Could you check a few things on this model? Use its own coordinates, in mm. A direction names the side the tool comes from. Give positions to 0.01 mm unless a question says otherwise; leave off trailing zeros. Loops run counter-clockwise (first coordinate to the right, second up) from the corner with the lowest first, then second, coordinate; pieces in that order, holes last.
1. Imagine slicing it at D-D (y = 100). List the corners of the cut face in (x, z) for me, plus the area to 3 significant figures.
2. For faces 5 (the flat face through (-25.4, 66, 13)), 6 (the flat face through (25.4, 67, 13)), 7 (the flat face through (0, 27.5, 13)), which set-ups out of +Z, -Z, +X, -X, +Y, -Y let a thin tool reach every point of the face, with its end or its side?
3. For P1, Ø10, axis at y = 59, z = 18, coming from the -X side; P2, Ø3, axis at x = 7.5, z = 13.5, coming from the -Y side; P3, Ø5, axis at x = 17, y = 13.5, coming from the +Z side; P4, Ø0.8, axis at y = 27, z = 11.5, coming from the +X side, each with a flat end and sliding along its axis, tell me the tip position at first contact or that it passes through.
4. I need wall thicknesses on line 1 along X through (y, z) = (0, 14.25); line 2 along Y through (x, z) = (9, 8); line 3 along Y through (x, z) = (-11.25, 9.5). Which ranges of each line are inside material? Lowest first, please.
5. Thinking about a two-plate mould opening in Y: for faces 1 (the flat face through (0, 109.08, 13)), 2 (the cylindrical face through (-13.748, 65.11, 12.878)), 3 (the flat face through (0, 54, 0)), 4 (the flat face through (2.5, 26, 13)), which applies, +Y half, -Y half, draft (parallel to the pull), parting line (faces both ways), or undercut?
6. Imagine slicing it at B-B (x = 0). List the corners of the cut face in (y, z) for me.
7. Imagine slicing it at A-A (y = 0). List the corners of the cut face in (x, z) for me.
8. Imagine slicing it at C-C (z = 18.5). List the corners of the cut face in (x, y) for me.
```python
from build123d import *

# Parameters (mm, degrees)
SKETCH1_R           = 25
BOSS_EXTRUDE1_DEPTH = 25.4
SKETCH2_W           = 5
SKETCH2_H           = 27.5
CUT_EXTRUDE1_DEPTH  = 118.339581594
SKETCH3_R           = 2.5
CUT_EXTRUDE2_DEPTH  = 118.339581594


with BuildPart() as part:
    # Sketch1 → Boss-Extrude1 (new body)
    with BuildSketch(Plane.XY):
        with BuildLine():
            Line((-25.4, 24.079867109), (-25.4, 109.079867109))
            Line((-25.4, 109.079867109), (25.4, 109.079867109))
            Line((25.4, 109.079867109), (25.4, 24.079867109))
            ThreePointArc((25.4, 24.079867109), (0, -35), (-25.4, 24.079867109))
        make_face()
        Circle(SKETCH1_R, mode=Mode.SUBTRACT)
    extrude(amount=BOSS_EXTRUDE1_DEPTH)

    # Sketch2 → Cut-Extrude1 (cut, through all)
    with BuildSketch(Plane.XY.offset(25.4)):
        with Locations((0, 13.75)):
            Rectangle(SKETCH2_W, SKETCH2_H)
    extrude(amount=-CUT_EXTRUDE1_DEPTH, mode=Mode.SUBTRACT)

    # Sketch3 → Cut-Extrude2 (cut, through all)
    with BuildSketch(Plane.XY.offset(25.4)):
        with Locations((-11.25, 100)):
            Circle(SKETCH3_R)
        with Locations((11.25, 100)):
            Circle(SKETCH3_R)
        with Locations((11.25, 65)):
            Circle(SKETCH3_R)
        with Locations((-11.25, 65)):
            Circle(SKETCH3_R)
    extrude(amount=-CUT_EXTRUDE2_DEPTH, mode=Mode.SUBTRACT)


solid = part.part
```
Derived:
1. outline: (-25.4, 0) - (-13.75, 0) - (-13.75, 25.4) - (-25.4, 25.4) - close; (-8.75, 0) - (8.75, 0) - (8.75, 25.4) - (-8.75, 25.4) - close; (13.75, 0) - (25.4, 0) - (25.4, 25.4) - (13.75, 25.4) - close
1. area: 1,040 mm2
2. face 5: +Z, -Z, -X, +Y
2. face 6: +Z, -Z, +X, +Y
2. face 7: +Z, -Z
3. P1: stops at x = -25.4
3. P2: stops at y = -34.48
3. P3: passes through
3. P4: stops at x = 25.4
4. line 1: x = -35 to -25, 25 to 35
4. line 2: y = -33.82 to -23.32, 23.32 to 63.91, 66.09 to 98.91, 101.09 to 109.08
4. line 3: y = -33.14 to -22.33, 22.33 to 62.5, 67.5 to 97.5, 102.5 to 109.08
5. face 1: +Y half
5. face 2: undercut
5. face 3: draft
5. face 4: undercut
6. outline: (-35, 0) - (-25, 0) - (-25, 25.4) - (-35, 25.4) - close; (27.5, 0) - (109.08, 0) - (109.08, 25.4) - (27.5, 25.4) - close
7. outline: (-35, 0) - (-25, 0) - (-25, 25.4) - (-35, 25.4) - close; (25, 0) - (35, 0) - (35, 25.4) - (25, 25.4) - close
8. outline: (-25.4, 24.08) arc R35 ccw (long way) to (25.4, 24.08) - (25.4, 109.08) - (-25.4, 109.08) - close; hole circle Ø5 at (-11.25, 65); hole circle Ø5 at (-11.25, 100); hole (-2.5, 24.87) arc R25 ccw (long way) to (2.5, 24.87) - (2.5, 27.5) - (-2.5, 27.5) - close; hole circle Ø5 at (11.25, 65); hole circle Ø5 at (11.25, 100)
